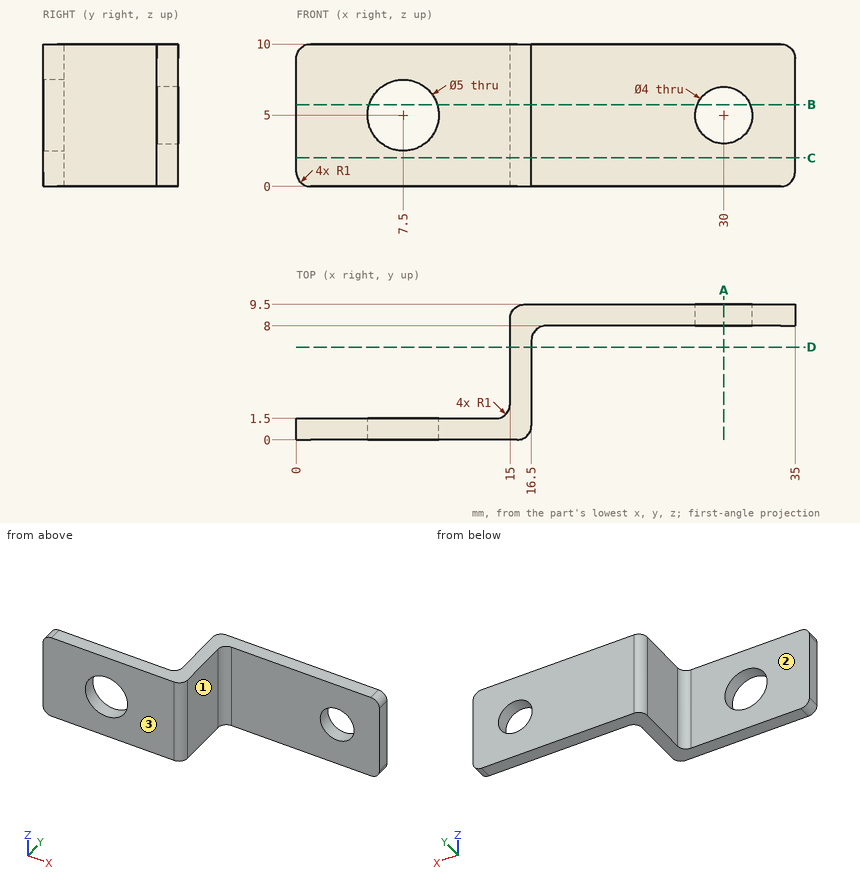
Source: three-view drawing plus pictorial views. Frame: mm from the lowest corner of the part. A direction names the side the tool comes from. Round coordinates to 2 decimals unless told otherwise and drop trailing zeros. Loops run counter-clockwise (first coordinate to the right, second up) from the corner with the lowest first, then second, coordinate; pieces in that order, holes last.
Q1. Material intervals for L1, parallel to X at y = 8.4, z = 5; L2, parallel to Y at x = 23, z = 8.75; L3, parallel to X at y = 8.25, z = 3.25, sorted ascending.
Q2. Section C-C on z = 2. Return loops of the section in (x, y), plus the area to 3 significant figures.
Q3. Section A-A on x = 30. Return loops of the section in (y, z), plus the area to 3 significant figures.
Q4. Access query for the marked faces 1, 2 and 3. Directions: +Z, -Z, +X, -X, +Y, -Y. A direction counts if a zero-diameter tool reaches every point of the face in a straight line with its end or side. Return the directions, or none.
Q5. Section B-B on z = 5.75. Return loops of the section in (x, y).
Q6. Pin query (flat end, axial travel): P1, Ø2, axis at x = 15, z = 3.5, coming from the +Y side; P2, Ø1.5, axis at y = 8.5, z = 8, coming from the -X side; P3, Ø3, axis at y = 5, z = 2.5, coming from the +X side; P4, Ø3, axis at x = 5.5, z = 5, coming from the +Y side. Return the tip coordinate at first contact, or that it passes through.
Q7. Section D-D on y = 6.5. Return loops of the section in (x, z), plus the area to 3 significant figures.
Evaluation:
1. L1: x = 15 to 28, 32 to 35
1. L2: y = 8 to 9.5
1. L3: x = 15 to 29.03, 30.97 to 35
2. outline: (0, 0) - (15.5, 0) arc R1 ccw to (16.5, 1) - (16.5, 7) arc R1 cw to (17.5, 8) - (35, 8) - (35, 9.5) - (16, 9.5) arc R1 ccw to (15, 8.5) - (15, 2.5) arc R1 cw to (14, 1.5) - (0, 1.5) - close
2. area: 64.5 mm2
3. outline: (8, 0) - (9.5, 0) - (9.5, 3) - (8, 3) - close; (8, 7) - (9.5, 7) - (9.5, 10) - (8, 10) - close
3. area: 9.00 mm2
4. face 1: +Z, -Z, +X, -Y
4. face 2: +Z, -Z, -X, +Y
4. face 3: +Z, -Z, +X, -X, -Y
5. outline: (0, 0) - (5.12, 0) - (5.12, 1.5) - (0, 1.5) - close; (9.88, 0) - (15.5, 0) arc R1 ccw to (16.5, 1) - (16.5, 7) arc R1 cw to (17.5, 8) - (28.15, 8) - (28.15, 9.5) - (16, 9.5) arc R1 ccw to (15, 8.5) - (15, 2.5) arc R1 cw to (14, 1.5) - (9.88, 1.5) - close; (31.85, 8) - (35, 8) - (35, 9.5) - (31.85, 9.5) - close
6. P1: stops at y = 9.5
6. P2: stops at x = 15
6. P3: stops at x = 16.5
6. P4: stops at y = 1.5
7. outline: (15, 0) - (16.5, 0) - (16.5, 10) - (15, 10) - close
7. area: 15.0 mm2
